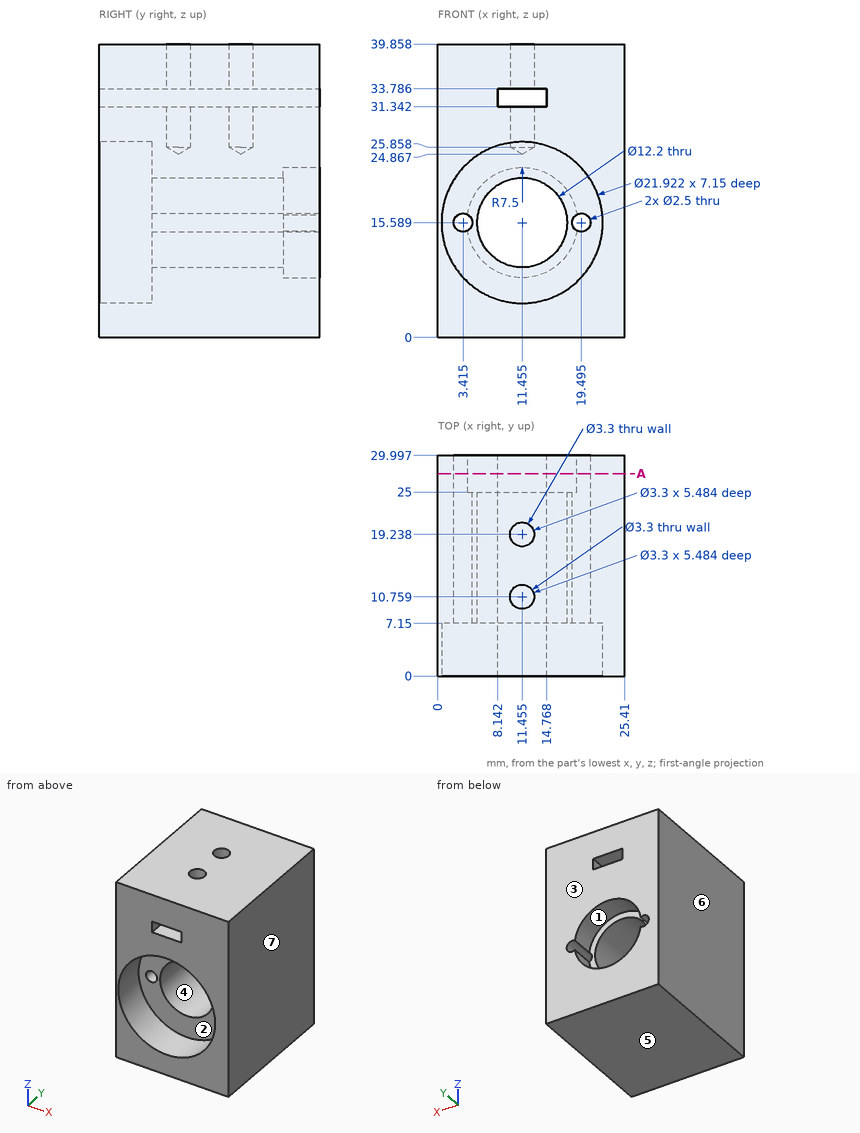
The figure shows three views and two pictorial views of one solid part (mm, origin at its lowest corner). Answer the questions. A direction names the side the tool comes from. Give positions to 0.01 mm unless a question says otherwise; leave off trailing zeros. Answer in a Markdown table with one row per item.
(1) Section A-A (y = 27.5) is taken. State how many separate pieces and enclosed holes the cut face has, and give its area (3 significant figures).
Results list:
| item | result |
|---|---|
| separate pieces | 1 |
| enclosed holes | 2 |
| area | 812 mm² |
(2) A tool of negligible diameter and unlimited length cuts with its end or side. For the marked faces 1, 2 and 3, from which of +Z, -Z, +X, -X, +Y, -Y can it reach the whole face along a straight path? Write none if from no direction.
Results list:
| item | result |
|---|---|
| face 1 | +Y |
| face 2 | -Y |
| face 3 | +Z, -Z, +X, -X, +Y |
(3) For a pull along X with two mould halves and no side action, classify the marked faces 4, 5, 6 and 7 as pulls with the +X half, pulls with the -X half, needs draft (parallel to the pull), parting line crosses it, or undercut.
Results list:
| item | result |
|---|---|
| face 4 | undercut |
| face 5 | needs draft |
| face 6 | pulls with the -X half |
| face 7 | pulls with the +X half |
(4) Flat-ended cylindrical pins translate along their axes: pin 1 Ø3 at (x, y) = (11.455, 19.238) entering from +Z; pin 2 Ø12 at (x, z) = (12, 16) entering from +Y; pin 3 Ø4 at (x, z) = (19.495, 15.589) entering from -Y; pin 4 Ø4.5 at (x, z) = (9, 16) entering from +Y. Find the tip coordinate at first contact, or state that the pin passes through.
Results list:
| item | result |
|---|---|
| pin 1 | stops at z = 25.77 |
| pin 2 | stops at y = 25 |
| pin 3 | stops at y = 7.15 |
| pin 4 | passes through |
(5) Consider L1, parallel to Z at x = 14.5, y = 3.5 (1 decimal); L2, parallel to Z at x = 8.5, y = 20.25 (1 decimal); L3, parallel to Y at x = 6, z = 20. Determine where each line is inside the solid, lowest interval first. Write a range as [from, to].
Results list:
| item | result |
|---|---|
| L1 | z = [0, 5.1], [26.1, 31.3], [33.8, 39.9] |
| L2 | z = [0, 10.3], [20.9, 31.3], [33.8, 39.9] |
| L3 | y = [7.15, 25] |
